Model file for the job. Use its own axes, mm. Face numbers are marked on the shaded views. A direction names the side the tool comes from. Round coordinates to 2 decimals unless told otherwise and drop trailing zeros. Write each loop counter-clockwise with the first axis right and the second up, starting at its lowest first coordinate (ties: lowest second). Pieces come first, ordered by that corner, then holes. Notation, with made-up numbers: (82.25, 22.25) - (100.25, 22.25) arc R19 cw to (100.25, 57.25) - close; hole circle Ø1 at (18, 84). An arc over 180 degrees is marked (long way). One line per item, written item: value.
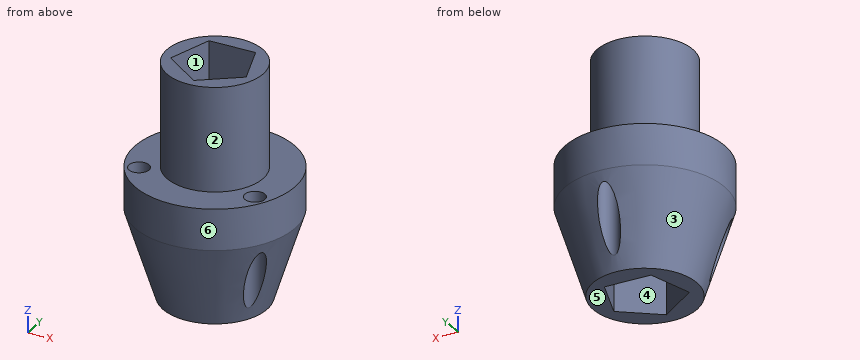
from build123d import *

# Parameters (mm, degrees)
SKETCH2_R                      = 9
BOSS_EXTRUDE1_DEPTH            = 19.5
CUT_EXTRUDE1_DEPTH             = 49.576640477
F_3_8_3_8_DIAMETER_HOLE1_D     = 3.8
F_3_8_3_8_DIAMETER_HOLE1_DEPTH = 24.2


with BuildPart() as part:
    # Sketch1 → Revolve1 (revolve)
    with BuildSketch(Plane.XZ, mode=Mode.PRIVATE) as revolve1_sk:
        Polygon((15, 24.2), (0, 24.2), (0, 0), (9.754545455, 0), (15, 16.485714286), align=None)
    revolve(revolve1_sk.sketch.rotate(Axis((0, 0, 24.2), (0, 0, -1)), 180), axis=Axis((0, 0, 24.2), (0, 0, -1)))

    # Sketch2 → Boss-Extrude1 (add)
    with BuildSketch(Plane.XY.offset(24.2)):
        Circle(SKETCH2_R)
    extrude(amount=BOSS_EXTRUDE1_DEPTH)

    # Sketch3 → Cut-Extrude1 (cut, through all)
    with BuildSketch(Plane(origin=(0, 0, 0), x_dir=(-1, 0, 0), z_dir=(0, 0, -1))):
        Polygon((0, -7.416407865), (7.053423028, -2.291796068), (4.359255168, 6), (-4.359255168, 6), (-7.053423028, -2.291796068), align=None)
    extrude(amount=-CUT_EXTRUDE1_DEPTH, mode=Mode.SUBTRACT)

    # Ø3.8 (3.8) Diameter Hole1
    with Locations(Plane.XY.offset(24.2)):
        with Locations((10.825317547, -6.25), (-10.825317547, -6.25), (0, 12.5)):
            Hole(F_3_8_3_8_DIAMETER_HOLE1_D / 2, depth=F_3_8_3_8_DIAMETER_HOLE1_DEPTH)


solid = part.part
1. Mould opens along X. For the marked faces 4, 5 and 6 say: released by +X, released by -X, zero draft, split by the parting line, or undercut.
Report:
face 4: undercut
face 5: zero draft
face 6: split by the parting line
2. Drop flat-ended pins along their axis: pin 1 (3 mm diameter, centred on x = -10.83, y = -6.25, fed in from -Z); pin 2 (2.5 mm diameter, centred on x = -2, z = 15, fed in from -Y); pin 3 (3 mm diameter, centred on y = -4.5, z = 10, fed in from +X); pin 4 (6 mm diameter, centred on x = 10.83, y = -6.25, fed in from +Z). Give the stop position or say it passes through.
Report:
pin 1: through
pin 2: y = -14.82
pin 3: x = 12.82
pin 4: z = 24.2
3. Band-saw the part on A-A on y = 0. Write the cut outline in (x, z).
Report:
outline: (-15, 16.49) - (-9.75, 0) - (-6.31, 0) - (-6.31, 43.7) - (-9, 43.7) - (-9, 24.2) - (-15, 24.2) - close; (6.31, 0) - (9.75, 0) - (15, 16.49) - (15, 24.2) - (9, 24.2) - (9, 43.7) - (6.31, 43.7) - close
4. Wall check: probe 1 along Z at (x, y) = (-1.5, -9); probe 2 along Y at (x, z) = (-12.5, 22); probe 3 along Y at (x, z) = (-3.5, 2). Give the ranges that are in metal, low to high. Write a range as [from, to].
Report:
probe 1: [0, 24.2]
probe 2: [-8.29, -7.15], [-5.35, 8.29]
probe 3: [-9.78, -4.87], [6, 9.78]
5. Band-saw the part on C-C on y = -6.25. State how many separate pieces and enclosed holes the cut face has, plus the area to 3 significant figures.
Report:
separate pieces: 4
enclosed holes: 0
area: 556 mm²
6. Band-saw the part on B-B on z = 32. Write the cut outline in (x, y), plus the area to 3 significant figures.
Report:
outline: circle Ø18 at (0, 0); hole (-7.05, -2.29) - (0, -7.42) - (7.05, -2.29) - (4.36, 6) - (-4.36, 6) - close
area: 124 mm²
7. Band-saw the part on D-D on z = 4.5. Write the cut outline in (x, y), plus the area to 3 significant figures.
Report:
outline: (-10.27, -4.43) arc R1.9 cw to (-8.97, -6.68) arc R11.19 ccw to (8.97, -6.68) arc R1.9 cw to (10.27, -4.43) arc R11.19 ccw to (1.3, 11.11) arc R1.9 cw to (-1.3, 11.11) arc R11.19 ccw to start; hole (-7.05, -2.29) - (0, -7.42) - (7.05, -2.29) - (4.36, 6) - (-4.36, 6) - close
area: 259 mm²
8. Tool access for the marked faces 1, 2 and 3: list every direction of +Z, -Z, +X, -X, +Y, -Y with a clear straight run to the whole face (end or side of a thin tool).
Report:
face 1: +Z, -Z
face 2: +Z
face 3: -Z
